```python
from build123d import *

# Parameters (mm, degrees)
SKETCH1_W           = 212
SKETCH1_H           = 162
SKETCH1_W_2         = 200
SKETCH1_H_2         = 150
BOSS_EXTRUDE1_DEPTH = 100
SKETCH1_4_W         = 200
SKETCH1_4_H         = 150
BOSS_EXTRUDE2_DEPTH = 4
SKETCH2_W           = 206
SKETCH2_H           = 156
SKETCH2_W_2         = 200
SKETCH2_H_2         = 150
CUT_EXTRUDE1_DEPTH  = 10
SKETCH3_W           = 15
SKETCH3_H           = 150
CUT_EXTRUDE2_DEPTH  = 200
BOSS_EXTRUDE3_DEPTH = 200
BOSS_EXTRUDE4_DEPTH = 150
SKETCH6_R           = 3
SKETCH6_R_2         = 1.4
BOSS_EXTRUDE5_DEPTH = 3
CUT_EXTRUDE3_START  = -4
SKETCH6_3_R         = 1.4
CUT_EXTRUDE3_DEPTH  = 4
SKETCH6_5_R         = 4.5
CUT_EXTRUDE4_DEPTH  = 6
BOSS_EXTRUDE6_START = 10
SKETCH6_6_R         = 5.75
SKETCH6_6_R_2       = 4.5
BOSS_EXTRUDE6_DEPTH = 10
FILLET1_R           = 3
SKETCH6_8_R         = 1.4
SKETCH6_8_W         = 7
SKETCH6_8_H         = 7
BOSS_EXTRUDE7_DEPTH = 15


with BuildPart() as part:
    # Sketch1 → Boss-Extrude1 (new body)
    with BuildSketch(Plane.XY):
        Rectangle(SKETCH1_W, SKETCH1_H)
        Rectangle(SKETCH1_W_2, SKETCH1_H_2, mode=Mode.SUBTRACT)
    extrude(amount=BOSS_EXTRUDE1_DEPTH)

    # Sketch1_4 → Boss-Extrude2 (add)
    with BuildSketch(Plane.XY):
        Rectangle(SKETCH1_4_W, SKETCH1_4_H)
    extrude(amount=BOSS_EXTRUDE2_DEPTH)

    # Sketch2 → Cut-Extrude1 (cut)
    with BuildSketch(Plane.XY.offset(100)):
        Rectangle(SKETCH2_W, SKETCH2_H)
        Rectangle(SKETCH2_W_2, SKETCH2_H_2, mode=Mode.SUBTRACT)
    extrude(amount=-CUT_EXTRUDE1_DEPTH, mode=Mode.SUBTRACT)

    # Sketch3 → Cut-Extrude2 (cut)
    with BuildSketch(Plane(origin=(106, 0, 0), x_dir=(0, 0, -1), z_dir=(1, 0, 0))):
        with Locations((-50, 0)):
            Rectangle(SKETCH3_W, SKETCH3_H)
    extrude(amount=-CUT_EXTRUDE2_DEPTH, mode=Mode.SUBTRACT)

    # Sketch4 → Boss-Extrude3 (add)
    with BuildSketch(Plane.ZY.offset(-100)):
        Polygon((42.5, 75), (42.5, 70), (32.5, 75), align=None)
        Polygon((32.5, -75), (42.5, -75), (42.5, -70), align=None)
    extrude(amount=BOSS_EXTRUDE3_DEPTH)

    # Sketch5 → Boss-Extrude4 (add)
    with BuildSketch(Plane.XZ.offset(-75)):
        Polygon((100, 9), (-100, 4), (100, 4), align=None)
    extrude(amount=BOSS_EXTRUDE4_DEPTH)

    # Sketch6 → Boss-Extrude5 (add)
    # profile 1 of 12: a face of its own
    with BuildSketch(Plane.ZY.offset(106)):
        with Locations(Location((57.5, 31, 0), (0, 0, 270))):
            Circle(SKETCH6_R)
        with Locations(Location((57.5, 31, 0), (0, 0, 90))):
            Circle(SKETCH6_R_2, mode=Mode.SUBTRACT)
    # profile 2 of 12: a face of its own
    with BuildSketch(Plane.ZY.offset(106)):
        with Locations(Location((42.5, 31, 0), (0, 0, 90))):
            Circle(SKETCH6_R)
        with Locations(Location((42.5, 31, 0), (0, 0, 270))):
            Circle(SKETCH6_R_2, mode=Mode.SUBTRACT)
    # profile 3 of 12: a face of its own
    with BuildSketch(Plane.ZY.offset(106)):
        with Locations(Location((57.5, -13, 0), (0, 0, 270))):
            Circle(SKETCH6_R)
        with Locations(Location((57.5, -13, 0), (0, 0, 90))):
            Circle(SKETCH6_R_2, mode=Mode.SUBTRACT)
    # profile 4 of 12: a face of its own
    with BuildSketch(Plane.ZY.offset(106)):
        with Locations(Location((42.5, -13, 0), (0, 0, 90))):
            Circle(SKETCH6_R)
        with Locations(Location((42.5, -13, 0), (0, 0, 270))):
            Circle(SKETCH6_R_2, mode=Mode.SUBTRACT)
    # profile 5 of 12: a face of its own
    with BuildSketch(Plane.ZY.offset(106)):
        with Locations(Location((67.5, -32, 0), (0, 0, 90))):
            Circle(SKETCH6_R)
        with Locations(Location((67.5, -32, 0), (0, 0, 270))):
            Circle(SKETCH6_R_2, mode=Mode.SUBTRACT)
    # profile 6 of 12: a face of its own
    with BuildSketch(Plane.ZY.offset(106)):
        with Locations(Location((67.5, -51, 0), (0, 0, 90))):
            Circle(SKETCH6_R)
        with Locations(Location((67.5, -51, 0), (0, 0, 270))):
            Circle(SKETCH6_R_2, mode=Mode.SUBTRACT)
    # profile 7 of 12: a face of its own
    with BuildSketch(Plane.ZY.offset(106)):
        with Locations(Location((32.5, -51, 0), (0, 0, 270))):
            Circle(SKETCH6_R)
        with Locations(Location((32.5, -51, 0), (0, 0, 90))):
            Circle(SKETCH6_R_2, mode=Mode.SUBTRACT)
    # profile 8 of 12: a face of its own
    with BuildSketch(Plane.ZY.offset(106)):
        with Locations(Location((32.5, -32, 0), (0, 0, 270))):
            Circle(SKETCH6_R)
        with Locations(Location((32.5, -32, 0), (0, 0, 90))):
            Circle(SKETCH6_R_2, mode=Mode.SUBTRACT)
    # profile 9 of 12: a face of its own
    with BuildSketch(Plane.ZY.offset(106)):
        with Locations(Location((14.5, 31, 0), (0, 0, 90))):
            Circle(SKETCH6_R)
        with Locations(Location((14.5, 31, 0), (0, 0, 270))):
            Circle(SKETCH6_R_2, mode=Mode.SUBTRACT)
    # profile 10 of 12: a face of its own
    with BuildSketch(Plane.ZY.offset(106)):
        with Locations(Location((14.5, -13, 0), (0, 0, 90))):
            Circle(SKETCH6_R)
        with Locations(Location((14.5, -13, 0), (0, 0, 270))):
            Circle(SKETCH6_R_2, mode=Mode.SUBTRACT)
    # profile 11 of 12: a face of its own
    with BuildSketch(Plane.ZY.offset(106)):
        with Locations(Location((85.5, -13, 0), (0, 0, 270))):
            Circle(SKETCH6_R)
        with Locations(Location((85.5, -13, 0), (0, 0, 90))):
            Circle(SKETCH6_R_2, mode=Mode.SUBTRACT)
    # profile 12 of 12: a face of its own
    with BuildSketch(Plane.ZY.offset(106)):
        with Locations(Location((85.5, 31, 0), (0, 0, 270))):
            Circle(SKETCH6_R)
        with Locations(Location((85.5, 31, 0), (0, 0, 90))):
            Circle(SKETCH6_R_2, mode=Mode.SUBTRACT)
    extrude(amount=BOSS_EXTRUDE5_DEPTH)

    # Sketch6_3 → Cut-Extrude3 (cut)
    with BuildSketch(Plane.ZY.offset(106).offset(CUT_EXTRUDE3_START)):
        with Locations(Location((57.5, 31, 0), (0, 0, 270))):
            Circle(SKETCH6_3_R)
        with Locations(Location((42.5, 31, 0), (0, 0, 270))):
            Circle(SKETCH6_3_R)
        with Locations(Location((42.5, -13, 0), (0, 0, 270))):
            Circle(SKETCH6_3_R)
        with Locations(Location((57.5, -13, 0), (0, 0, 270))):
            Circle(SKETCH6_3_R)
        with Locations(Location((67.5, -32, 0), (0, 0, 270))):
            Circle(SKETCH6_3_R)
        with Locations(Location((32.5, -32, 0), (0, 0, 270))):
            Circle(SKETCH6_3_R)
        with Locations(Location((32.5, -51, 0), (0, 0, 270))):
            Circle(SKETCH6_3_R)
        with Locations(Location((67.5, -51, 0), (0, 0, 270))):
            Circle(SKETCH6_3_R)
    extrude(amount=CUT_EXTRUDE3_DEPTH, mode=Mode.SUBTRACT)

    # Sketch6_5 → Cut-Extrude4 (cut)
    with BuildSketch(Plane.ZY.offset(106)):
        with Locations(Location((11, -60, 0), (0, 0, 270))):
            Circle(SKETCH6_5_R)
    extrude(amount=-CUT_EXTRUDE4_DEPTH, mode=Mode.SUBTRACT)

    # Sketch6_6 → Boss-Extrude6 (add)
    with BuildSketch(Plane.ZY.offset(106).offset(BOSS_EXTRUDE6_START)):
        with Locations(Location((11, -60, 0), (0, 0, 90))):
            Circle(SKETCH6_6_R)
        with Locations(Location((11, -60, 0), (0, 0, 270))):
            Circle(SKETCH6_6_R_2, mode=Mode.SUBTRACT)
    extrude(amount=-BOSS_EXTRUDE6_DEPTH)

    # Fillet1
    fillet1_edges = [part.edges().sort_by_distance(p)[0] for p in [
        (-100, -55.5, 11),
    ]]
    fillet(fillet1_edges, radius=FILLET1_R)

    # Sketch6_8 → Boss-Extrude7 (add)
    # profile 1 of 4: a face of its own
    with BuildSketch(Plane.ZY.offset(106)):
        Polygon((93, 88), (83, 81), (100, 81), (100, 88), align=None)
        with Locations(Location((96.5, 84.5, 0), (0, 0, 270))):
            Circle(SKETCH6_8_R, mode=Mode.SUBTRACT)
    # profile 2 of 4: a face of its own
    with BuildSketch(Plane.ZY.offset(106)):
        with Locations((3.5, 84.5)):
            Rectangle(SKETCH6_8_W, SKETCH6_8_H)
        with Locations(Location((3.5, 84.5, 0), (0, 0, 270))):
            Circle(SKETCH6_8_R, mode=Mode.SUBTRACT)
    # profile 3 of 4: a face of its own
    with BuildSketch(Plane.ZY.offset(106)):
        Polygon((100, -81), (83, -81), (93, -88), (100, -88), align=None)
        with Locations(Location((96.5, -84.5, 0), (0, 0, 270))):
            Circle(SKETCH6_8_R, mode=Mode.SUBTRACT)
    # profile 4 of 4: a face of its own
    with BuildSketch(Plane.ZY.offset(106)):
        with Locations((3.5, -84.5)):
            Rectangle(SKETCH6_8_W, SKETCH6_8_H)
        with Locations(Location((3.5, -84.5, 0), (0, 0, 270))):
            Circle(SKETCH6_8_R, mode=Mode.SUBTRACT)
    extrude(amount=-BOSS_EXTRUDE7_DEPTH)


solid = part.part
```
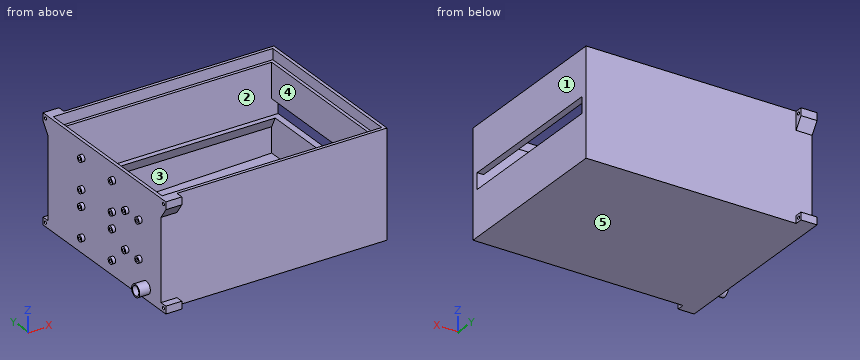
Here's how the part is built. I have some questions about the finished solid (model axes, mm). Face numbers are marked on the shaded views. A direction names the side the tool comes from. Give positions to 0.01 mm unless a question says otherwise; leave off trailing zeros. Order: outer loops, then holes, each group sorted by start corner. A loop starts at its lowest first (then second) coordinate and runs counter-clockwise, first axis right, second up. Notation, with made-up numbers: (-31, -23.75) -> (-19, -23.75) arc R33 cw to (-19, 12.25) -> close; hole circle Ø11 at (57.5, 20). An arc over 180 degrees is marked (long way). Use CSV: the item, a comma, the result in double quotes. Start each with the question number.
Item 1: Suppose I cut it at D-D (x = -21). List the corners of the cut face in (y, z) for me (3 decimals), and give its area (3 significant figures).
Item 2: If I drill on probe 1 along Y at (x, z) = (39, 32); probe 2 along Z at (x, y) = (-101.5, 84.5); probe 3 along X at (y, z) = (58.5, 67.5), over which ranges is the centre line in solid material (lowest first)? Write a range as [from, to].
Item 3: Suppose I cut it at A-A (y = 50). List the corners of the cut face in (x, z) for me.
Item 4: On a 3-axis mill with a long thin cutter (end or side, diameter ignored), from which of +Z, -Z, +X, -X, +Y, -Y can I reach the whole of each face in a straight line? I mean the marked faces 3, 4 and 5. Say none if no direction works.
Item 5: Thinking about a two-plate mould opening in Y: for the marked faces 1 and 2, which applies, pulls with the +Y half, pulls with the -Y half, needs draft (parallel to the pull), parting line crosses it, or undercut?
Item 6: Suppose I cut it at B-B (z = 48). List the corners of the cut face in (x, y) for me.
Item 7: Suppose I cut it at C-C (x = 54). List the corners of the cut face in (y, z) for me.
Item 8: I'm going to push flat-ended pins straight in: P1, Ø1, axis at x = -41.5, y = -29.5, coming from the +Z side (3 decimals); P2, Ø3, axis at x = 57, z = 40.5, coming from the -Y side; P3, Ø12, axis at x = 44, z = 40, coming from the +Y side. Where does each tip first touch, or does it pass through?
Answer block:
1,outline,"(-81, 0) -> (81, 0) -> (81, 100) -> (78, 100) -> (78, 90) -> (75, 90) -> (75, 42.5) -> (70, 42.5) -> (75, 32.5) -> (75, 5.975) -> (-75, 5.975) -> (-75, 32.5) -> (-70, 42.5) -> (-75, 42.5) -> (-75, 90) -> (-78, 90) -> (-78, 100) -> (-81, 100) -> close"
1,area,"2,090 mm^2"
2,probe 1,"y = [-81, -75], [75, 81]"
2,probe 2,"z = [0, 2.1], [4.9, 7], [88, 95.1], [97.9, 100]"
2,probe 3,"x = [-106, -100], [100, 106]"
3,outline,"(-106, 0) -> (106, 0) -> (106, 42.5) -> (100, 42.5) -> (100, 9) -> (-100, 4) -> (-100, 90) -> (-103, 90) -> (-103, 100) -> (-106, 100) -> close; (100, 57.5) -> (106, 57.5) -> (106, 100) -> (103, 100) -> (103, 90) -> (100, 90) -> close"
4,face 3,"none"
4,face 4,"+Z"
4,face 5,"-Z, +X, -X, +Y, -Y"
5,face 1,"needs draft"
5,face 2,"undercut"
6,outline,"(-106, -81) -> (106, -81) -> (106, -75) -> (-100, -75) -> (-100, 75) -> (106, 75) -> (106, 81) -> (-106, 81) -> close"
7,outline,"(-81, 0) -> (81, 0) -> (81, 100) -> (78, 100) -> (78, 90) -> (75, 90) -> (75, 42.5) -> (70, 42.5) -> (75, 32.5) -> (75, 7.85) -> (-75, 7.85) -> (-75, 32.5) -> (-70, 42.5) -> (-75, 42.5) -> (-75, 90) -> (-78, 90) -> (-78, 100) -> (-81, 100) -> close"
8,P1,"stops at z = 5.475"
8,P2,"stops at y = -81"
8,P3,"stops at y = 81"
